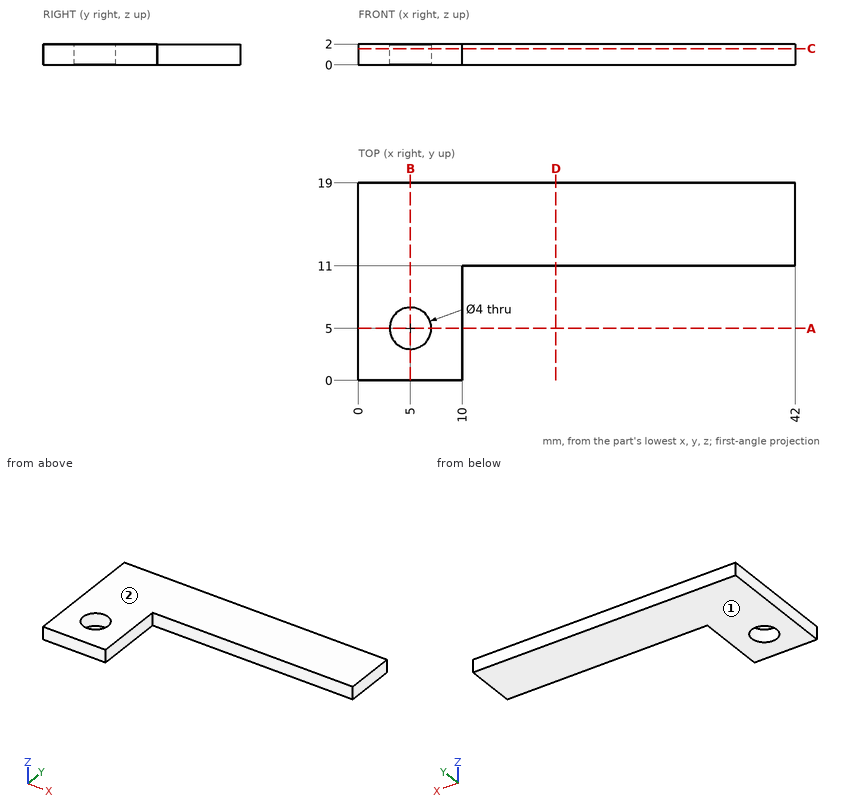
Check sheet for the drawn part. Datum: minimum x, y, z corner. Units: mm. Give positions to 0.01 mm unless a question says otherwise; leave off trailing zeros. Write each loop counter-clockwise with the first axis right and the second up, starting at its lowest first coordinate (ties: lowest second). Pieces come first, ordered by that corner, then holes. Notation, with made-up numbers: (-27, 51.5) - (3, 51.5) arc R16 cw to (3, 55.5) - close; hole circle Ø6 at (23, 70). An arc over 180 degrees is marked (long way). Put each result on its own line as item: value.
1. Sectioned sample at D-D, the plane x = 19. Enter the section's corners in (y, z), plus the area to 3 significant figures.
Ans:
outline: (11, 0) - (19, 0) - (19, 2) - (11, 2) - close
area: 16.0 mm²
2. Sectioned sample at A-A, the plane y = 5. Enter the section's corners in (x, z).
Ans:
outline: (0, 0) - (3, 0) - (3, 2) - (0, 2) - close; (7, 0) - (10, 0) - (10, 2) - (7, 2) - close
3. Draft check along Z on the marked faces 1 and 2. Enter one of: +Z half, -Z half, draft (parallel to the pull), parting line (faces both ways), or undercut.
Ans:
face 1: -Z half
face 2: +Z half
4. Sectioned sample at C-C, the plane z = 1.55. Enter the section's corners in (x, y).
Ans:
outline: (0, 0) - (10, 0) - (10, 11) - (42, 11) - (42, 19) - (0, 19) - close; hole circle Ø4 at (5, 5)
5. Sectioned sample at B-B, the plane x = 5. Enter the section's corners in (y, z).
Ans:
outline: (0, 0) - (3, 0) - (3, 2) - (0, 2) - close; (7, 0) - (19, 0) - (19, 2) - (7, 2) - close
6. Thickness scan on line 1 (Y direction, x = 5, z = 0.5); line 2 (X direction, y = 9, z = 1.15); line 3 (X direction, y = 6.5, z = 1.6). Record the ranges inside material, lowest first.
Ans:
line 1: y = 0 to 3, 7 to 19
line 2: x = 0 to 10
line 3: x = 0 to 3.68, 6.32 to 10
